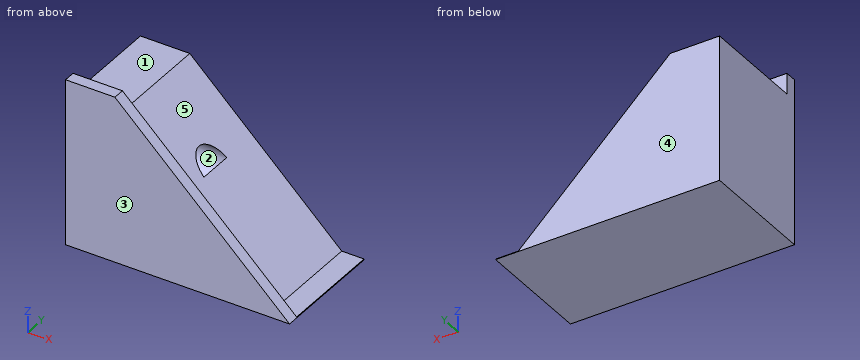
```python
from build123d import *

# Parameters (mm, degrees)
F1_DEPTH = 50.8
F3_DEPTH = 45.72
F4_R     = 7.799938
F5_DEPTH = 25.4


with BuildPart() as f1:
    # F0 (on Front) → F1 (new body)
    with BuildSketch(Plane.XZ):
        Polygon((-27.354645, 36.2239), (-48.827574, 36.2239), (-48.827574, -36.2239), (48.640851, -36.2239), align=None)
    extrude(amount=F1_DEPTH)

    # F2 (on Front) → F3 (cut)
    with BuildSketch(Plane.XZ):
        Polygon((-27.354645, 36.597338), (-48.827574, 36.597338), (-48.827574, 27.138793), (-27.354645, 27.138793), (38.744636, -36.037177), (48.640851, -36.037177), align=None)
    extrude(amount=F3_DEPTH, mode=Mode.SUBTRACT)

    # F4 (on Right) → F5 (cut)
    with BuildSketch(Plane.YZ):
        with Locations((-25.300711, 0)):
            Circle(F4_R)
    extrude(amount=-F5_DEPTH, mode=Mode.SUBTRACT)


solid = f1.part
```
Geometry check sheet. Reference: the model listing, model coordinates, mm. Face numbers are marked on the shaded views. A direction names the side the tool comes from. Round coordinates to 2 decimals unless told otherwise and drop trailing zeros. Order: outer loops, then holes, each group sorted by start corner. A loop starts at its lowest first (then second) coordinate and runs counter-clockwise, first axis right, second up. Notation, with made-up numbers: (3.5, 83.5) - (32.5, 83.5) arc R21 ccw to (32.5, 98.5) - close; hole circle Ø4 at (24.5, 89.5). An arc over 180 degrees is marked (long way). Use a Markdown table: item, result. Add a question column.
(1) Sectioned sample at C-C, the plane y = -35. Enter the section's corners in (x, z), and give its area (3 significant figures).
(2) Sectioned sample at A-A, the plane x = -36. Enter the section's corners in (y, z), and give its area (3 significant figures).
(3) Depth check by flat-ended pin: pin 1 (2 mm diameter, centred on y = -26.5, z = 16, fed in from +X); pin 2 (10.5 mm diameter, centred on x = -38, y = -11.5, fed in from +Z); pin 3 (17 mm diameter, centred on y = -25, z = 2, fed in from +X). Enter the tip coordinate at first touch or a pass-through.
(4) Tool access check on the marked faces 4 and 5. Record the directions out of +Z, -Z, +X, -X, +Y, -Y that give a thin tool (end or side, any length) a straight path to the whole face; none if there is none.
(5) Sectioned sample at D-D, the plane x = -16.5. Enter the section's corners in (y, z).
(6) Sectioned sample at B-B, the plane z = -6.5. Enter the section's corners in (x, y).
(7) Release check for a two-part mould opening along Y. For the marked faces 1, 2 and 3 record: pulls with the +Y half, pulls with the -Y half, needs draft (parallel to the pull), parting line crosses it, or undercut.
(8) Material ranges on line 1 along Y through (x, z) = (-6.5, 0); line 2 along Z through (x, y) = (-41.5, -40.5); line 3 along Z through (x, y) = (-18, -24), recorded low to high. Write a range as [from, to].
Answers below:
| question | item | result |
|---|---|---|
| 1 | outline | (-48.83, -36.22) - (48.64, -36.22) - (48.44, -36.04) - (38.74, -36.04) - (-27.35, 27.14) - (-48.83, 27.14) - close |
| 1 | area | 3,460 mm² |
| 2 | outline | (-50.8, -36.22) - (0, -36.22) - (0, 27.14) - (-45.72, 27.14) - (-45.72, 36.22) - (-50.8, 36.22) - close |
| 2 | area | 3,260 mm² |
| 3 | pin 1 | x = -14.65 |
| 3 | pin 2 | z = 27.14 |
| 3 | pin 3 | x = 7.84 |
| 4 | face 4 | +Z, -Z, +X, -X, +Y |
| 4 | face 5 | +Z, +X, +Y |
| 5 | outline | (-50.8, -36.22) - (0, -36.22) - (0, 16.76) - (-45.72, 16.76) - (-45.72, 25.88) - (-50.8, 25.88) - close; hole circle Ø15.6 at (-25.3, 0) |
| 6 | outline | (-48.83, -50.8) - (17.46, -50.8) - (17.46, -45.72) - (7.84, -45.72) - (7.84, 0) - (-48.83, 0) - close; hole (-25.4, -29.61) - (0, -29.61) - (0, -20.99) - (-25.4, -20.99) - close |
| 7 | face 1 | needs draft |
| 7 | face 2 | undercut |
| 7 | face 3 | pulls with the -Y half |
| 8 | line 1 | [-50.8, -33.1], [-17.5, 0] |
| 8 | line 2 | [-36.22, 27.14] |
| 8 | line 3 | [-36.22, -7.69], [7.69, 18.2] |
